CAD build for the part. Positions are in the model's coordinates, mm. Give positions to 0.01 mm unless a question says otherwise; leave off trailing zeros. Order: outer loops, then holes, each group sorted by start corner. A loop starts at its lowest first (then second) coordinate and runs counter-clockwise, first axis right, second up.
Item 1: Band-saw the part on A-A on z = 787.4. Give the cut face in (x, y), plus the area to 3 significant figures.
Item 2: Band-saw the part on B-B on x = -22. Give the cut face in (y, z).
Item 3: Band-saw the part on C-C on z = 332.5. Give the cut face in (x, y), plus the area to 3 significant figures.
Item 4: Band-saw the part on D-D on z = 25.4. Give the cut face in (x, y), plus the area to 3 significant figures.
Item 5: Wall check: L1, parallel to Y at x = -17.75, z = 482; L2, parallel to X at y = -20, z = 699; L3, parallel to Y at x = -12.25, z = 787.4. Give the ranges that are in metal, low to high.
Autodesk Inventor part; units mm, degrees
ref_plane "YZ Plane" through (0, 0, 0) normal (1, 0, 0) x (0, 1, 0)
ref_plane "XZ Plane" through (0, 0, 0) normal (0, 1, 0) x (-1, 0, 0)
ref_plane "XY Plane" through (0, 0, 0) normal (0, 0, 1) x (1, 0, 0)
sketch "Sketch1" plane through (0, 0, 0) normal (0, 0, 1) x (1, 0, 0)
  line L0 (-35.3228, 16.049) -> (-9.9228, 16.049)
  line L1 (-9.9228, 16.049) -> (-9.9228, -34.751)
  line L2 (-9.9228, -34.751) -> (-35.3228, -34.751)
  line L3 (-35.3228, -34.751) -> (-35.3228, 16.049)
  line L4 (-13.0978, 12.874) -> (-32.1478, 12.874)
  line L5 (-32.1478, 12.874) -> (-32.1478, -31.576)
  line L6 (-32.1478, -31.576) -> (-13.0978, -31.576)
  line L7 (-13.0978, -31.576) -> (-13.0978, 12.874)
  point P0 (0, 0)
  dimension "d0" = 25.4
  dimension "d1" = 50.8
  dimension "d2" = 3.175
extrude "Extrusion1" add sketch "Sketch1" along normal blind 965.2
sketch "Sketch2" plane through (-35.3228, -34.751, 0) normal (-1, 0, 0) x (0, 0, 1)
  line L0 (0, 0) -> (0, 50.8) construction
  line L1 (0, 25.4) -> (25.4, 25.4) construction
  circle A0 centre (25.4, 25.4) radius 12.7
  point P0 (0, 34.751)
  dimension "d5" = 25.4
  dimension "d9" = 25.4
extrude "Extrusion2" cut sketch "Sketch2" against normal blind 254
sketch "Sketch3" plane through (-35.3228, -34.751, 0) normal (-1, 0, 0) x (0, 0, 1)
  line L0 (965.2, 50.8) -> (965.2, 0) construction
  line L1 (965.2, 25.4) -> (787.4, 25.4) construction
  circle A0 centre (787.4, 25.4) radius 14.2875
  point P0 (0, 34.751)
  dimension "d10" = 177.8
  dimension "d11" = 28.575
extrude "Extrusion3" cut sketch "Sketch3" against normal blind 25.4
sketch "Sketch4" plane through (-35.3228, -34.751, 0) normal (-1, 0, 0) x (0, 0, 1)
  line L0 (965.2, 50.8) -> (965.2, 0) construction
  line L1 (965.2, 25.4) -> (406.4, 25.4) construction
  circle A0 centre (406.4, 25.4) radius 14.2875
  point P0 (0, 34.751)
  dimension "d14" = 558.8
  dimension "d15" = 28.575
extrude "Extrusion4" cut sketch "Sketch4" against normal blind 25.4
sketch "Sketch5" plane through (-35.3228, -34.751, 0) normal (-1, 0, 0) x (0, 0, 1)
  circle A0 centre (406.4, 25.4) radius 14.2875 construction
  line L0 (406.4, 25.4) -> (388.4395, 7.4395) construction
  line L1 (406.4, 25.4) -> (431.8, 25.4) construction
  line L2 (406.4, 25.4) -> (424.3605, 43.3605) construction
  circle A1 centre (388.4395, 7.4395) radius 2.032
  circle A2 centre (424.3605, 43.3605) radius 2.032
  point P0 (0, 34.751)
  dimension "d18" = 25.4
  dimension "d19" = 135
  dimension "d20" = 25.4
  dimension "d21" = 4.064
  dimension "d22" = 4.064
extrude "Extrusion5" cut sketch "Sketch5" against normal blind 25.4
properties part number "34.48in Arm Bea"
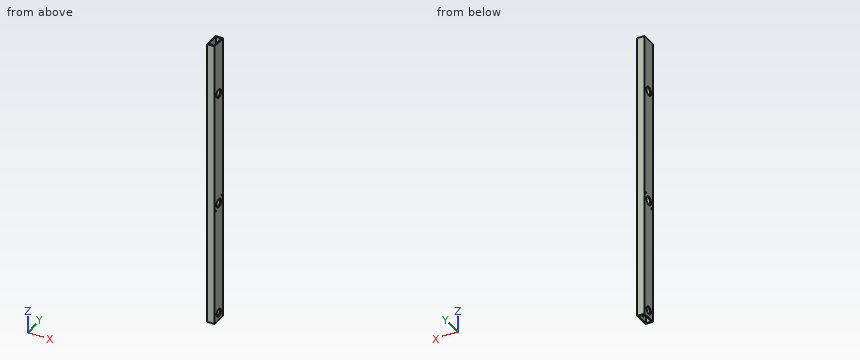
The answers:
1. outline: (-35.32, -34.75) - (-9.92, -34.75) - (-9.92, -23.64) - (-13.1, -23.64) - (-13.1, -31.58) - (-32.15, -31.58) - (-32.15, -23.64) - (-35.32, -23.64) - close; (-35.32, 4.94) - (-32.15, 4.94) - (-32.15, 12.87) - (-13.1, 12.87) - (-13.1, 4.94) - (-9.92, 4.94) - (-9.92, 16.05) - (-35.32, 16.05) - close
1. area: 262 mm2
2. outline: (-34.75, 0) - (-31.58, 0) - (-31.58, 965.2) - (-34.75, 965.2) - close; (12.87, 0) - (16.05, 0) - (16.05, 965.2) - (12.87, 965.2) - close
3. outline: (-35.32, -34.75) - (-9.92, -34.75) - (-9.92, 16.05) - (-35.32, 16.05) - close; hole (-32.15, -31.58) - (-13.1, -31.58) - (-13.1, 12.87) - (-32.15, 12.87) - close
3. area: 444 mm2
4. outline: (-35.32, -34.75) - (-9.92, -34.75) - (-9.92, -22.05) - (-13.1, -22.05) - (-13.1, -31.58) - (-32.15, -31.58) - (-32.15, -22.05) - (-35.32, -22.05) - close; (-35.32, 3.35) - (-32.15, 3.35) - (-32.15, 12.87) - (-13.1, 12.87) - (-13.1, 3.35) - (-9.92, 3.35) - (-9.92, 16.05) - (-35.32, 16.05) - close
4. area: 282 mm2
5. L1: y = -34.75 to -31.58, 12.87 to 16.05
5. L2: x = -35.32 to -32.15, -13.1 to -9.92
5. L3: y = -34.75 to -23.64, 4.94 to 16.05
